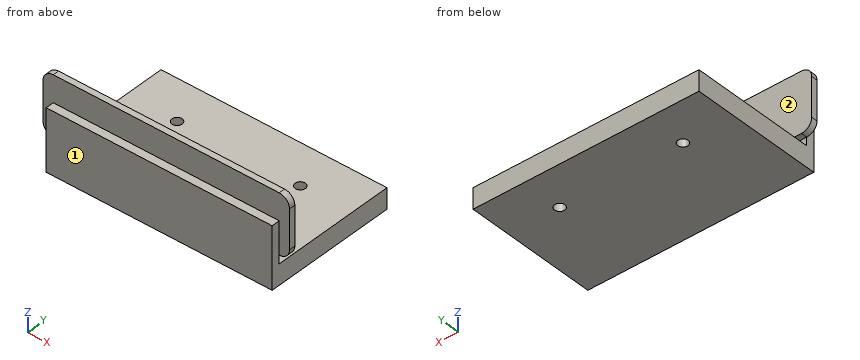
```python
from build123d import *

# Parameters (mm, degrees)
ESQUISSE1_W             = 110
ESQUISSE1_H             = 65
BOSS_EXTRU_1_DEPTH      = 10
ESQUISSE2_W             = 110
ESQUISSE2_H             = 4
BOSS_EXTRU_2_DEPTH      = 20
ESQUISSE3_W             = 120
ESQUISSE3_H             = 29
BOSS_EXTRU_3_DEPTH      = 3
CONG_1_R                = 5
ESQUISSE4_R             = 2.5
ENL_V_MAT_EXTRU_1_DEPTH = 76.797427397


with BuildPart() as part:
    # Esquisse1 → Boss.-Extru.1 (new body)
    with BuildSketch(Plane.XY):
        Rectangle(ESQUISSE1_W, ESQUISSE1_H)
    extrude(amount=BOSS_EXTRU_1_DEPTH)

    # Esquisse2 → Boss.-Extru.2 (add)
    with BuildSketch(Plane.XY.offset(10)):
        with Locations((0, -30.5)):
            Rectangle(ESQUISSE2_W, ESQUISSE2_H)
    extrude(amount=BOSS_EXTRU_2_DEPTH)

    # Esquisse3 → Boss.-Extru.3 (add)
    with BuildSketch(Plane(origin=(0, -28.5, 0), x_dir=(1, 0, 0), z_dir=(0, 1, 0))):
        with Locations((0, -28.5)):
            Rectangle(ESQUISSE3_W, ESQUISSE3_H)
    extrude(amount=BOSS_EXTRU_3_DEPTH)

    # Congé1
    cong_1_edges = [part.edges().sort_by_distance(p)[0] for p in [
        (60, -27, 14),
        (60, -27, 43),
        (-60, -27, 43),
        (-60, -27, 14),
    ]]
    fillet(cong_1_edges, radius=CONG_1_R)

    # Esquisse4 → Enlèv. mat.-Extru.1 (cut, through all)
    with BuildSketch(Plane.XY.offset(10)):
        with Locations((-30, 12.5)):
            Circle(ESQUISSE4_R)
        with Locations((30, 12.5)):
            Circle(ESQUISSE4_R)
    extrude(amount=-ENL_V_MAT_EXTRU_1_DEPTH, mode=Mode.SUBTRACT)


solid = part.part
```
Could you check a few things on this model? Use its own coordinates, in mm. Face numbers are marked on the shaded views. A direction names the side the tool comes from. Round coordinates to 2 decimals unless told otherwise and drop trailing zeros. Loops run counter-clockwise (first coordinate to the right, second up) from the corner with the lowest first, then second, coordinate; pieces in that order, holes last. Notation, with made-up numbers: (65.25, 80.25) - (95.25, 80.25) arc R7 cw to (95.25, 87.25) - close; hole circle Ø4 at (64, -6). An arc over 180 degrees is marked (long way). Answer in a Markdown table with one row per item. Add a question column.
(1) If we section it at C-C (x = 10): Please give me the cut outline in (y, z), plus the area to 3 significant figures.
(2) If we section it at A-A (y = 12.5): Please give me the cut outline in (x, z), plus the area to 3 significant figures.
(3) I need wall thicknesses on line 1 along Y through (x, z) = (-30, 5); line 2 along Z through (x, y) = (16.5, 19); line 3 along Y through (x, z) = (-26, 31). Which ranges of each line are inside material? Lowest first, please.
(4) If we section it at B-B (x = -30): Please give me the cut outline in (y, z), plus the area to 3 significant figures.
(5) I'm going to push flat-ended pins straight in: pin 1 (4.5 mm diameter, centred on x = -30, y = 12.5, fed in from +Z); pin 2 (2 mm diameter, centred on x = -5.5, y = -30.5, fed in from +Z); pin 3 (6 mm diameter, centred on x = 41, y = -16, fed in from +Z); pin 4 (23 mm diameter, centred on x = 10.5, z = 27, fed in from +Y). Where does each tip first touch, or does it pass through?
(6) For the marked faces 1 and 2, which set-ups out of +Z, -Z, +X, -X, +Y, -Y let a thin tool reach every point of the face, with its end or its side?
(7) If we section it at D-D (z = 32): Please give me the cut outline in (x, y).
Model answer:
| question | item | result |
|---|---|---|
| 1 | outline | (-32.5, 0) - (32.5, 0) - (32.5, 10) - (-28.5, 10) - (-28.5, 14) - (-25.5, 14) - (-25.5, 43) - (-28.5, 43) - (-28.5, 30) - (-32.5, 30) - close |
| 1 | area | 817 mm² |
| 2 | outline | (-55, 0) - (-32.5, 0) - (-32.5, 10) - (-55, 10) - close; (-27.5, 0) - (27.5, 0) - (27.5, 10) - (-27.5, 10) - close; (32.5, 0) - (55, 0) - (55, 10) - (32.5, 10) - close |
| 2 | area | 1,000 mm² |
| 3 | line 1 | y = -32.5 to 10, 15 to 32.5 |
| 3 | line 2 | z = 0 to 10 |
| 3 | line 3 | y = -28.5 to -25.5 |
| 4 | outline | (-32.5, 0) - (10, 0) - (10, 10) - (-28.5, 10) - (-28.5, 14) - (-25.5, 14) - (-25.5, 43) - (-28.5, 43) - (-28.5, 30) - (-32.5, 30) - close; (15, 0) - (32.5, 0) - (32.5, 10) - (15, 10) - close |
| 4 | area | 767 mm² |
| 5 | pin 1 | passes through |
| 5 | pin 2 | stops at z = 30 |
| 5 | pin 3 | stops at z = 10 |
| 5 | pin 4 | stops at y = -25.5 |
| 6 | face 1 | +Z, -Z, +X, -X, -Y |
| 6 | face 2 | +Z, +X, -X, +Y |
| 7 | outline | (-60, -28.5) - (60, -28.5) - (60, -25.5) - (-60, -25.5) - close |
